Job drawing, mm, ordinate dimensions from the low corner. One solid piece. A direction names the side the tool comes from. Round coordinates to 2 decimals unless told otherwise and drop trailing zeros. Loops run counter-clockwise (first coordinate to the right, second up) from the corner with the lowest first, then second, coordinate; pieces in that order, holes last. Notation, with made-up numbers: M 75.25,21.5 L 91.25,21.5 A12 cw 91.25,32.5 Z; hole C 59.5,-10 d2. An arc over 180 degrees is marked long. Use a Markdown table: item, result. Add a question column.
(1) Band-saw the part on A-A, the plane z = 1.65. Write the cut outline in (x, y) (1 decimal).
(2) Which spindle directions (+Z, -Z, +X, -X, +Y, -Y) get a long thin tool onto all of the face, cutting with end or side? Do the marked faces 1 and 2. Say none if no direction does.
(3) Band-saw the part on C-C, the plane x = 42.5. Write the cut outline in (y, z), and give its area (3 significant figures).
(4) Two-plate mould, pull along Y, no slides. Class the marked faces 3, 4, 5 and 6: released by +Y, released by -Y, zero draft, split by the parting line, or undercut.
(5) Band-saw the part on B-B, the plane y = 18. Write the cut outline in (x, z).
(6) Flat gauge pins, fed straight in: P1, Ø2.5, axis at y = 53.5, z = 2.5, coming from the +X side; P2, Ø8, axis at x = 12, y = 26.5, coming from the -Z side. Where does each tip first touch, or does it go through?
(7) Wall check: L1, parallel to Y at x = 3, z = 2.2 (1 decimal); L2, parallel to X at y = 62, z = 1.1; L3, parallel to Y at x = 18, z = 1.2. Give the ranges that are in metal, low to high.
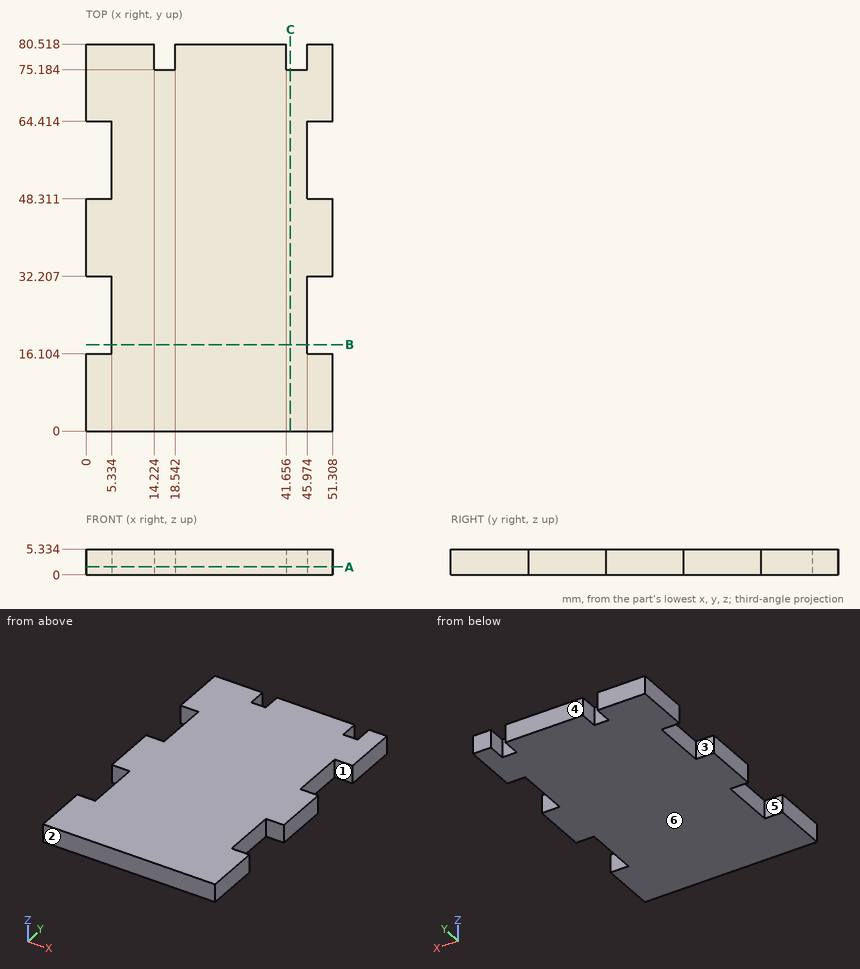
Return value:
| question | item | result |
|---|---|---|
| 1 | outline | M 0,0 L 51.3,0 L 51.3,16.1 L 46,16.1 L 46,32.2 L 51.3,32.2 L 51.3,48.3 L 46,48.3 L 46,64.4 L 51.3,64.4 L 51.3,80.5 L 46,80.5 L 46,75.2 L 41.7,75.2 L 41.7,80.5 L 18.5,80.5 L 18.5,75.2 L 14.2,75.2 L 14.2,80.5 L 0,80.5 L 0,64.4 L 5.3,64.4 L 5.3,48.3 L 0,48.3 L 0,32.2 L 5.3,32.2 L 5.3,16.1 L 0,16.1 Z |
| 2 | face 1 | +Z, -Z, +X |
| 2 | face 2 | +Z, -Z, +X, -X, -Y |
| 3 | outline | M 0,0 L 75.18,0 L 75.18,5.33 L 0,5.33 Z |
| 3 | area | 401 mm^2 |
| 4 | face 3 | undercut |
| 4 | face 4 | released by +Y |
| 4 | face 5 | undercut |
| 4 | face 6 | zero draft |
| 5 | outline | M 5.33,0 L 45.97,0 L 45.97,5.33 L 5.33,5.33 Z |
| 6 | P1 | x = 45.97 |
| 6 | P2 | z = 0 |
| 7 | L1 | 0 to 16.1, 32.2 to 48.3, 64.4 to 80.5 |
| 7 | L2 | 5.33 to 45.97 |
| 7 | L3 | 0 to 75.18 |
